Geometry check sheet. Reference: the model listing, model coordinates, mm. Face numbers are marked on the shaded views. A direction names the side the tool comes from. Give positions to 0.01 mm unless a question says otherwise; leave off trailing zeros. Write each loop counter-clockwise with the first axis right and the second up, starting at its lowest first coordinate (ties: lowest second). Pieces come first, ordered by that corner, then holes. Notation, with made-up numbers: (76.25, 76.5) - (81.25, 76.5) arc R24 ccw to (81.25, 88.5) - close; hole circle Ø2 at (87, 84). An arc over 180 degrees is marked (long way). One line per question, with ' | ' between items. Start each with the question number.
Q1. Section check D-D on y = -26.5. Record the boundary of the cut face in (x, z), and give its area (3 significant figures).
Q2. Gauge pin test, flat ends, axial feed: P1, Ø2, axis at x = -51, z = 20.5, coming from the -Y side; P2, Ø2, axis at x = -30.5, y = -33.5, coming from the +Z side; P3, Ø11, axis at x = -15.5, y = -5.5, coming from the -Z side. Record the tip position at first contact, or that the pin passes through.
Q3. Section check C-C on z = 35. Record the boundary of the cut face in (x, y).
Q4. Section check A-A on y = -40.5. Record the boundary of the cut face in (x, z).
Q5. Set-up check for the marked faces 1, 2, 3, 4 and 5: record each of +Z, -Z, +X, -X, +Y, -Y from which the full face is reachable in a straight line by a thin tool's end or side.
Q6. Thickness scan on L1, parallel to X at y = -25, z = 32.5; L2, parallel to Y at x = -33.5, z = 11; L3, parallel to Z at x = -34, y = -18. Record the ranges inside material, lowest first. Write a range as [from, to].
```python
from build123d import *

# Parameters (mm, degrees)
SKETCH2_W                 = 70
SKETCH2_H                 = 35
BOSS_EXTRUDE2_DEPTH       = 40
SKETCH3_W                 = 28.105894453
SKETCH3_H                 = 27.971945797
CUT_EXTRUDE1_DEPTH        = 10
SKETCH4_R                 = 10
CUT_EXTRUDE2_DEPTH        = 3
SKETCH5_R                 = 10
CUT_EXTRUDE3_DEPTH        = 3
SKETCH6_R                 = 10
BOSS_EXTRUDE3_DEPTH       = 3
BOSS_EXTRUDE3_DEPTH_BACK  = 3
SKETCH7_R                 = 10
BOSS_EXTRUDE5_DEPTH       = 6
SKETCH8_R                 = 2
CUT_EXTRUDE5_DEPTH        = 46
SKETCH9_R                 = 2
BOSS_EXTRUDE8_DEPTH       = 0.0001
BOSS_EXTRUDE8_DEPTH_BACK  = 46.0001
SKETCH10_R                = 10
BOSS_EXTRUDE9_DEPTH       = 3
BOSS_EXTRUDE9_DEPTH_BACK  = 3
SKETCH11_R                = 10
BOSS_EXTRUDE10_DEPTH      = 3
BOSS_EXTRUDE10_DEPTH_BACK = 3
SKETCH12_R                = 2
CUT_EXTRUDE6_DEPTH        = 46
SKETCH13_R                = 2
BOSS_EXTRUDE11_DEPTH      = 0.001
BOSS_EXTRUDE11_DEPTH_BACK = 46.001
BOSS_EXTRUDE12_DEPTH      = 28
SKETCH18_R                = 4
CUT_EXTRUDE11_DEPTH       = 10
SKETCH19_R                = 5.5
BOSS_EXTRUDE13_DEPTH      = 0.001


with BuildPart() as part:
    # Sketch2 → Boss-Extrude2 (new body)
    with BuildSketch(Plane.XY):
        with Locations((-35, -17.5)):
            Rectangle(SKETCH2_W, SKETCH2_H)
    extrude(amount=BOSS_EXTRUDE2_DEPTH)

    # Sketch3 → Cut-Extrude1 (cut)
    with BuildSketch(Plane(origin=(0, 0, 0), x_dir=(1, 0, 0), z_dir=(0, 1, 0))):
        with Locations((-17.175677586, -20.094439992)):
            Rectangle(SKETCH3_W, SKETCH3_H)
    extrude(amount=-CUT_EXTRUDE1_DEPTH, mode=Mode.SUBTRACT)

    # Sketch4 → Cut-Extrude2 (cut)
    with BuildSketch(Plane.XY.offset(40)):
        with Locations((-15, -35)):
            Circle(SKETCH4_R)
        with Locations((-55, -35)):
            Circle(SKETCH4_R)
    extrude(amount=-CUT_EXTRUDE2_DEPTH, mode=Mode.SUBTRACT)

    # Sketch5 → Cut-Extrude3 (cut)
    with BuildSketch(Plane(origin=(0, 0, 0), x_dir=(-1, 0, 0), z_dir=(0, 0, -1))):
        with Locations((15, -35)):
            Circle(SKETCH5_R)
        with Locations((55, -35)):
            Circle(SKETCH5_R)
    extrude(amount=-CUT_EXTRUDE3_DEPTH, mode=Mode.SUBTRACT)

    # Sketch6 → Boss-Extrude3 (add, two sides)
    with BuildSketch(Plane.XY.offset(40)) as boss_extrude3_sk:
        with Locations((-55, -35)):
            Circle(SKETCH6_R)
    extrude(amount=BOSS_EXTRUDE3_DEPTH)
    extrude(boss_extrude3_sk.sketch, amount=-BOSS_EXTRUDE3_DEPTH_BACK)

    # Sketch7 → Boss-Extrude5 (add)
    with BuildSketch(Plane(origin=(0, 0, 3), x_dir=(-1, 0, 0), z_dir=(0, 0, -1))):
        with Locations((55, -35)):
            Circle(SKETCH7_R)
    extrude(amount=BOSS_EXTRUDE5_DEPTH)

    # Sketch8 → Cut-Extrude5 (cut)
    with BuildSketch(Plane(origin=(0, 0, -3), x_dir=(-1, 0, 0), z_dir=(0, 0, -1))):
        with Locations((55, -35)):
            Circle(SKETCH8_R)
    extrude(amount=-CUT_EXTRUDE5_DEPTH, mode=Mode.SUBTRACT)

    # Sketch9 → Boss-Extrude8 (add, two sides)
    with BuildSketch(Plane(origin=(0, 0, -3), x_dir=(-1, 0, 0), z_dir=(0, 0, -1))) as boss_extrude8_sk:
        with Locations((55, -35)):
            Circle(SKETCH9_R)
    extrude(amount=BOSS_EXTRUDE8_DEPTH)
    extrude(boss_extrude8_sk.sketch, amount=-BOSS_EXTRUDE8_DEPTH_BACK)

    # Sketch10 → Boss-Extrude9 (add, two sides)
    with BuildSketch(Plane.XY.offset(40)) as boss_extrude9_sk:
        with Locations((-15, -35)):
            Circle(SKETCH10_R)
    extrude(amount=BOSS_EXTRUDE9_DEPTH)
    extrude(boss_extrude9_sk.sketch, amount=-BOSS_EXTRUDE9_DEPTH_BACK)

    # Sketch11 → Boss-Extrude10 (add, two sides)
    with BuildSketch(Plane(origin=(0, 0, 0), x_dir=(-1, 0, 0), z_dir=(0, 0, -1))) as boss_extrude10_sk:
        with Locations((15, -35)):
            Circle(SKETCH11_R)
    extrude(amount=BOSS_EXTRUDE10_DEPTH)
    extrude(boss_extrude10_sk.sketch, amount=-BOSS_EXTRUDE10_DEPTH_BACK)

    # Sketch12 → Cut-Extrude6 (cut)
    with BuildSketch(Plane(origin=(0, 0, -3), x_dir=(-1, 0, 0), z_dir=(0, 0, -1))):
        with Locations((15, -35)):
            Circle(SKETCH12_R)
    extrude(amount=-CUT_EXTRUDE6_DEPTH, mode=Mode.SUBTRACT)

    # Sketch13 → Boss-Extrude11 (add, two sides)
    with BuildSketch(Plane(origin=(0, 0, -3), x_dir=(-1, 0, 0), z_dir=(0, 0, -1))) as boss_extrude11_sk:
        with Locations((15, -35)):
            Circle(SKETCH13_R)
    extrude(amount=BOSS_EXTRUDE11_DEPTH)
    extrude(boss_extrude11_sk.sketch, amount=-BOSS_EXTRUDE11_DEPTH_BACK)

    # Sketch14 → Boss-Extrude12 (add)
    with BuildSketch(Plane(origin=(0, 0, 34.080412891), x_dir=(-1, 0, 0), z_dir=(0, 0, -1))):
        Polygon((3.122730359, 0), (31.228624812, -10), (3.122730359, -10), align=None)
    extrude(amount=BOSS_EXTRUDE12_DEPTH)

    # Sketch18 → Cut-Extrude11 (cut)
    with BuildSketch(Plane(origin=(-0.350891722, 0.986212569, 0), x_dir=(0.942142791, 0.335211816, 0), z_dir=(-0.335211816, 0.942142791, 0))):
        with Locations((-16.374329601, -20.352535637)):
            Circle(SKETCH18_R)
    extrude(amount=-CUT_EXTRUDE11_DEPTH, mode=Mode.SUBTRACT)

    # Sketch19 → Boss-Extrude13 (add)
    with BuildSketch(Plane.ZY.offset(70)):
        with Locations((20, -5.5)):
            Circle(SKETCH19_R)
    extrude(amount=BOSS_EXTRUDE13_DEPTH)


solid = part.part
```
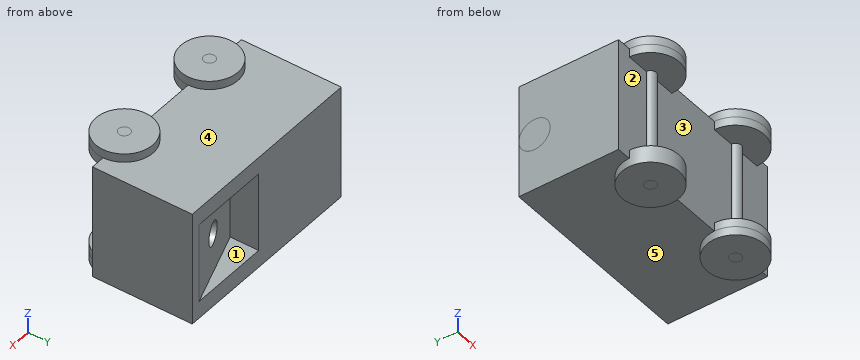
Working result:
1) outline: (-70, 0) - (-60.27, 0) - (-60.27, -3) - (-49.73, -3) - (-49.73, 0) - (-20.27, 0) - (-20.27, -3) - (-9.73, -3) - (-9.73, 0) - (0, 0) - (0, 40) - (-9.73, 40) - (-9.73, 43) - (-20.27, 43) - (-20.27, 40) - (-49.73, 40) - (-49.73, 43) - (-60.27, 43) - (-60.27, 40) - (-70, 40) - close | area: 2,930 mm2
2) P1: stops at y = -35 | P2: stops at z = 40 | P3: stops at z = 0
3) outline: (-70, -35) - (-57, -35) arc R2 ccw to (-53, -35) - (-17, -35) arc R2 ccw to (-13, -35) - (0, -35) - (0, 0) - (-70, 0) - close
4) outline: (-63.35, -3) - (-46.65, -3) - (-46.65, 3) - (-63.35, 3) - close; (-63.35, 37) - (-46.65, 37) - (-46.65, 43) - (-63.35, 43) - close; (-23.35, -3) - (-6.65, -3) - (-6.65, 3) - (-23.35, 3) - close; (-23.35, 37) - (-6.65, 37) - (-6.65, 43) - (-23.35, 43) - close
5) face 1: +Y | face 2: -X, -Y | face 3: -Y | face 4: +Z, +Y | face 5: -Z, +Y
6) L1: x = [-70, 0] | L2: y = [-35, 0] | L3: z = [0, 40]
